from build123d import *

# Parameters (mm, degrees)
SKETCH1_W           = 106
SKETCH1_H           = 142
BOSS_EXTRUDE1_DEPTH = 5
SKETCH2_W           = 90
SKETCH2_H           = 126
BOSS_EXTRUDE2_DEPTH = 5
SKETCH3_W           = 80
SKETCH3_H           = 116
CUT_EXTRUDE1_DEPTH  = 5
SKETCH4_W           = 25
SKETCH4_H           = 5
CUT_EXTRUDE2_DEPTH  = 5
FILLET1_R           = 5


with BuildPart() as part:
    # Sketch1 → Boss-Extrude1 (new body)
    with BuildSketch(Plane(origin=(0, 0, 0), x_dir=(1, 0, 0), z_dir=(0, 1, 0))):
        Rectangle(SKETCH1_W, SKETCH1_H)
    extrude(amount=BOSS_EXTRUDE1_DEPTH)

    # Sketch2 → Boss-Extrude2 (add)
    with BuildSketch(Plane.XZ):
        Rectangle(SKETCH2_W, SKETCH2_H)
    extrude(amount=BOSS_EXTRUDE2_DEPTH)

    # Sketch3 → Cut-Extrude1 (cut)
    with BuildSketch(Plane.XZ.offset(5)):
        Rectangle(SKETCH3_W, SKETCH3_H)
    extrude(amount=-CUT_EXTRUDE1_DEPTH, mode=Mode.SUBTRACT)

    # Sketch4 → Cut-Extrude2 (cut)
    with BuildSketch(Plane(origin=(45, 0, 0), x_dir=(0, 0, -1), z_dir=(1, 0, 0))):
        with Locations((0, -2.5)):
            Rectangle(SKETCH4_W, SKETCH4_H)
    extrude(amount=-CUT_EXTRUDE2_DEPTH, mode=Mode.SUBTRACT)

    # Fillet1
    fillet1_edges = [part.edges().sort_by_distance(p)[0] for p in [
        (-53, 5, 0),
        (0, 5, 71),
        (53, 5, 0),
        (53, 2.5, 71),
        (-53, 2.5, 71),
        (-53, 2.5, -71),
        (53, 2.5, -71),
        (0, 5, -71),
    ]]
    fillet(fillet1_edges, radius=FILLET1_R - 0.0001)  # a hair under: the kernel refuses the full size


solid = part.part
Could you check a few things on this model? Use its own coordinates, in mm. A direction names the side the tool comes from. Give positions to 0.01 mm unless a question says otherwise; leave off trailing zeros. Order: outer loops, then holes, each group sorted by start corner. A loop starts at its lowest first (then second) coordinate and runs counter-clockwise, first axis right, second up. Notation, with made-up numbers: (-20, 21.25) - (3, 21.25) arc R20 ccw to (3, 29.25) - close; hole circle Ø8 at (76, -13). An arc over 180 degrees is marked (long way). One line per item, written item: value. Start each with the question number.
1. If I drill on probe 1 along Z at (x, y) = (44.5, -0.25); probe 2 along Z at (x, y) = (-4, -2.5); probe 3 along X at (y, z) = (-3.5, -24.5), over which ranges is the centre line in solid material (lowest first)?
2. Imagine slicing it at A-A on y = -3. List the corners of the cut face in (x, z) for me.
3. Imagine slicing it at D-D on y = 3.5. List the corners of the cut face in (x, z) for me.
4. For faces 1 (the face through (45, -2, -38)), 2 (the face through (-1, -2, -63)), 3 (the face through (-1, -3, 58)), 4 (the face through (-45, -2, -1)), which set-ups out of +Z, -Z, +X, -X, +Y, -Y let a thin tool reach every point of the face, with its end or its side?
5. Thinking about a two-plate mould opening in X: for faces 5 (the face through (-40, -3, -1)), 6 (the face through (45, -2, 37)), 7 (the face through (-1, -2, 63)), which applies, +X half, -X half, draft (parallel to the pull), parting line (faces both ways), or undercut?
6. For P1, Ø4, axis at x = -0.5, z = -38, coming from the -Y side; P2, Ø5.5, axis at y = -3.5, z = -26, coming from the +X side; P3, Ø5, axis at x = 4, y = 3, coming from the -Z side, each with a flat end and sliding along its axis, tell me the tip position at first contact or that it passes through.
Values:
1. probe 1: -63 to -12.5, 12.5 to 63
1. probe 2: -63 to -58, 58 to 63
1. probe 3: -45 to -40, 40 to 45
2. outline: (-45, -63) - (45, -63) - (45, -12.5) - (40, -12.5) - (40, -58) - (-40, -58) - (-40, 58) - (40, 58) - (40, 12.5) - (45, 12.5) - (45, 63) - (-45, 63) - close
3. outline: (-51.57, -66) arc R3.57 ccw to (-48, -69.57) - (48, -69.57) arc R3.57 ccw to (51.57, -66) - (51.57, 66) arc R3.57 ccw to (48, 69.57) - (-48, 69.57) arc R3.57 ccw to (-51.57, 66) - close
4. face 1: +Z, -Z, +X, -Y
4. face 2: -Z, +X, -X, -Y
4. face 3: -Y
4. face 4: +Z, -Z, -X, -Y
5. face 5: undercut
5. face 6: +X half
5. face 7: draft
6. P1: y = 0
6. P2: x = 45
6. P3: z = -70.97
